Autodesk Inventor part; units mm, degrees
ref_plane "YZ Plane" through (0, 0, 0) normal (1, 0, 0) x (0, 1, 0)
ref_plane "XZ Plane" through (0, 0, 0) normal (0, 1, 0) x (-1, 0, 0)
ref_plane "XY Plane" through (0, 0, 0) normal (0, 0, 1) x (1, 0, 0)
sketch "Sketch1" plane through (0, 0, 0) normal (0, 1, 0) x (-1, 0, 0)
  line L0 (50, 50) -> (-50, 50)
  line L1 (-50, 50) -> (-50, -50)
  line L2 (-50, -50) -> (50, -50)
  line L3 (50, -50) -> (50, 50)
  line L4 (50, 50) -> (-50, -50) construction
  line L5 (-50, 50) -> (50, -50) construction
  line L6 (40, 40) -> (-40, 40)
  line L7 (-40, 40) -> (-40, -40)
  line L8 (-40, -40) -> (40, -40)
  line L9 (40, -40) -> (40, 40)
  line L10 (40, 40) -> (-40, -40) construction
  line L11 (-40, 40) -> (40, -40) construction
  point P0 (0, 0)
  dimension "d0" = 100
  dimension "d1" = 100
  dimension "d2" = 80
  dimension "d3" = 80
extrude "Extrusion1" add sketch "Sketch1" along normal blind 10
sketch "Sketch2" plane through (0, 10, 0) normal (0, 1, 0) x (1, 0, 0)
  line L0 (40, -40) -> (50, -40)
  line L1 (50, -40) -> (50, -50)
  line L2 (50, -50) -> (40, -50)
  line L3 (40, -50) -> (40, -40)
  line L4 (40, 40) -> (40, -40)
  line L5 (50, 50) -> (-50, 50)
  line L6 (40, 40) -> (50, 40)
  line L7 (50, 40) -> (50, 50)
  line L8 (50, 50) -> (40, 50)
  line L9 (40, 50) -> (40, 40)
  line L10 (-40, -40) -> (-40, 40)
  line L11 (-50, 50) -> (-50, -50)
  line L12 (-40, 40) -> (-50, 40)
  line L13 (-50, 40) -> (-50, 50)
  line L14 (-50, 50) -> (-40, 50)
  line L15 (-40, 50) -> (-40, 40)
  line L16 (40, -40) -> (-40, -40)
  line L17 (-40, -40) -> (-50, -40)
  line L18 (-50, -40) -> (-50, -50)
  line L19 (-50, -50) -> (-40, -50)
  line L20 (-40, -50) -> (-40, -40)
  point P0 (0, 0)
extrude "Extrusion2" add sketch "Sketch2" along normal blind 80 contours L0 L1 L2 L3 | L9 L5 L7 L6 | L20 L19 L11 L17 | L12 L11 L5 L15
sketch "Sketch3" plane through (0, 90, 0) normal (0, 1, 0) x (1, 0, 0)
  line L0 (-50, -50) -> (50, -50)
  line L1 (50, -50) -> (50, 50)
  line L2 (50, 50) -> (-50, 50)
  line L3 (-50, 50) -> (-50, -50)
  line L4 (-50, -50) -> (50, 50) construction
  line L5 (50, -50) -> (-50, 50) construction
  line L6 (-40, -40) -> (40, -40)
  line L7 (40, -40) -> (40, 40)
  line L8 (40, 40) -> (-40, 40)
  line L9 (-40, 40) -> (-40, -40)
  line L10 (-40, -40) -> (40, 40) construction
  line L11 (40, -40) -> (-40, 40) construction
  point P0 (0, 0)
  dimension "d8" = 100
  dimension "d9" = 100
  dimension "d10" = 80
  dimension "d11" = 80
extrude "Extrusion3" add sketch "Sketch3" along normal blind 10
properties part number "Hollow_Cube" material "ABS Plastic"
Check sheet for the modelled part. Datum: model origin and axes. Units: mm. A direction names the side the tool comes from. Round coordinates to 2 decimals unless told otherwise and drop trailing zeros. Loops run counter-clockwise (first coordinate to the right, second up) from the corner with the lowest first, then second, coordinate; pieces in that order, holes last. Notation, with made-up numbers: (-5, -8.75) -> (25, -8.75) arc R33 ccw to (25, 25.25) -> close; hole circle Ø10 at (81.5, 32.25). An arc over 180 degrees is marked (long way). Write item = value, one per line. Start each with the question number.
1) Sectioned sample at C-C, the plane y = 14. Record the cut outline in (x, z), plus the area to 3 significant figures.
2) Sectioned sample at A-A, the plane z = -42. Record the cut outline in (x, y).
3) Set-up check for faces 1 (the flat face through (40, 95, 1)), 2 (the flat face through (-1, 90, -45)), 3 (the flat face through (45, 10, 1)): record each of +Z, -Z, +X, -X, +Y, -Y from which the full face is reachable in a straight line by a thin tool's end or side.
4) Release check for a two-part mould opening along Z. For faces 4 (the flat face through (45, 49, 40)), 5 (the flat face through (45, 0, 1)), 6 (the flat face through (45, 49, -50)), 7 (the flat face through (-40, 95, -1)) record: released by +Z, released by -Z, zero draft, split by the parting line, or undercut.
5) Thickness scan on probe 1 along Z at (x, y) = (-13, 90.5). Record the ranges inside material, lowest first.
6) Sectioned sample at B-B, the plane x = 4. Record the cut outline in (y, z).
Results are:
q1.outline = (-50, -50) -> (-40, -50) -> (-40, -40) -> (-50, -40) -> close; (-50, 40) -> (-40, 40) -> (-40, 50) -> (-50, 50) -> close; (40, -50) -> (50, -50) -> (50, -40) -> (40, -40) -> close; (40, 40) -> (50, 40) -> (50, 50) -> (40, 50) -> close
q1.area = 400 mm^2
q2.outline = (-50, 0) -> (50, 0) -> (50, 100) -> (-50, 100) -> close; hole (-40, 10) -> (40, 10) -> (40, 90) -> (-40, 90) -> close
q3.face_1 = +Y, -Y
q3.face_2 = +Z, -Z
q3.face_3 = +X, -X
q4.face_4 = undercut
q4.face_5 = zero draft
q4.face_6 = released by -Z
q4.face_7 = undercut
q5.probe_1 = -50 to -40, 40 to 50
q6.outline = (0, -50) -> (10, -50) -> (10, -40) -> (0, -40) -> close; (0, 40) -> (10, 40) -> (10, 50) -> (0, 50) -> close; (90, -50) -> (100, -50) -> (100, -40) -> (90, -40) -> close; (90, 40) -> (100, 40) -> (100, 50) -> (90, 50) -> close
